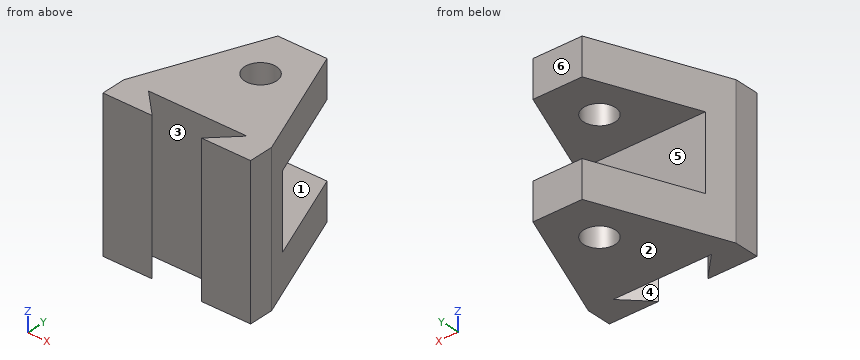
```python
from build123d import *

# Parameters (mm, degrees)
BOSS_EXTRUDE1_DEPTH = 60
SKETCH3_R           = 6.436223385
CUT_EXTRUDE1_DEPTH  = 61
SKETCH9_W           = 30
SKETCH9_H           = 40
CUT_EXTRUDE3_DEPTH  = 61


with BuildPart() as part:
    # Sketch2 → Boss-Extrude1 (new body)
    with BuildSketch(Plane.XY):
        Polygon((-30, -10), (-30, 0), (-10, 50), (10, 50), (30, 0), (30, -10), (10, -10), (20, 0), (-20, 0), (-10, -10), align=None)
    extrude(amount=BOSS_EXTRUDE1_DEPTH)

    # Sketch3 → Cut-Extrude1 (cut, through all)
    with BuildSketch(Plane.XY.offset(60)):
        with Locations((0, 30)):
            Circle(SKETCH3_R)
    extrude(amount=-CUT_EXTRUDE1_DEPTH, mode=Mode.SUBTRACT)

    # Sketch9 → Cut-Extrude3 (cut, through all)
    with BuildSketch(Plane(origin=(30, 0, 0), x_dir=(0, 0, -1), z_dir=(1, 0, 0))):
        with Locations((-30, 30)):
            Rectangle(SKETCH9_W, SKETCH9_H)
    extrude(amount=-CUT_EXTRUDE3_DEPTH, mode=Mode.SUBTRACT)


solid = part.part
```
Here's how the part is built. I have some questions about the finished solid (model axes, mm). Face numbers are marked on the shaded views. A direction names the side the tool comes from. Round coordinates to 2 decimals unless told otherwise and drop trailing zeros. Order: outer loops, then holes, each group sorted by start corner. A loop starts at its lowest first (then second) coordinate and runs counter-clockwise, first axis right, second up. Notation, with made-up numbers: M -38.75,88 L -16.75,88 A19 cw -16.75,119 Z; hole C 41,28.5 d9. An arc over 180 degrees is marked long. One line per question, with ' | ' between items.
1) For the marked faces 4, 5 and 6, which set-ups out of +Z, -Z, +X, -X, +Y, -Y let a thin tool reach every point of the face, with its end or its side?
Working result:
face 4: +Z, -Z | face 5: +X, -X, +Y | face 6: +Z, -Z, +X, -X, +Y
2) I need wall thicknesses on line 1 along Y through (x, z) = (0, 9); line 2 along Z through (x, y) = (21.5, 20.5); line 3 along Y through (x, z) = (-10.5, 34.5). Which ranges of each line are inside material? Lowest first, please.
Working result:
line 1: 0 to 23.56, 36.44 to 50 | line 2: 0 to 15, 45 to 60 | line 3: -10 to -9.5, 0 to 10
3) I want a section at A-A, the plane y = 42. Write out the boundary of the cut face in (x, z), then the cut area to 3 significant figures.
Working result:
outline: M -13.2,0 L 13.2,0 L 13.2,15 L -13.2,15 Z; M -13.2,45 L 13.2,45 L 13.2,60 L -13.2,60 Z | area: 792 mm²
4) I want a section at B-B, the plane x = 0. Write out the boundary of the cut face in (y, z), then the cut area to 3 significant figures.
Working result:
outline: M 0,0 L 23.56,0 L 23.56,15 L 10,15 L 10,45 L 23.56,45 L 23.56,60 L 0,60 Z; M 36.44,0 L 50,0 L 50,15 L 36.44,15 Z; M 36.44,45 L 50,45 L 50,60 L 36.44,60 Z | area: 1,410 mm²
5) For pin 1 Ø3 at (x, z) = (-22, 23.5) entering from +Y; pin 2 Ø8 at (y, z) = (8.5, 52) entering from -X; pin 3 Ø10 at (x, z) = (1, 9.5) entering from -Y, each with a flat end and sliding along its axis, tell me the tip position at first contact or that it passes through.
Working result:
pin 1: y = 10 | pin 2: x = -28.2 | pin 3: y = 0
6) I want a section at C-C, the plane y = 30. Write out the boundary of the cut face in (x, z), then the cut area to 3 significant figures.
Working result:
outline: M -18,0 L -6.44,0 L -6.44,15 L -18,15 Z; M -18,45 L -6.44,45 L -6.44,60 L -18,60 Z; M 6.44,0 L 18,0 L 18,15 L 6.44,15 Z; M 6.44,45 L 18,45 L 18,60 L 6.44,60 Z | area: 694 mm²
7) I want a section at D-D, the plane z = 46. Write out the boundary of the cut face in (x, y), then the cut area to 3 significant figures.
Working result:
outline: M -30,-10 L -10,-10 L -20,0 L 20,0 L 10,-10 L 30,-10 L 30,0 L 10,50 L -10,50 L -30,0 Z; hole C 0,30 d12.87 | area: 2,170 mm²
8) If we mould it in two halves opening along Z, with no side actions, what happens to the marked faces 1, 2 and 3? For each: +Z half, -Z half, draft (parallel to the pull), parting line (faces both ways), or undercut.
Working result:
face 1: undercut | face 2: -Z half | face 3: draft
